Design review of the part built by this model. Coordinates are the model's own, in mm. Face numbers are marked on the shaded views. A direction names the side the tool comes from. Give positions to 0.01 mm unless a question says otherwise; leave off trailing zeros. Write each loop counter-clockwise with the first axis right and the second up, starting at its lowest first coordinate (ties: lowest second). Pieces come first, ordered by that corner, then holes.
```python
from build123d import *

# Parameters (mm, degrees)
BOTTOM_SKETCH_W                   = 101.6
BOTTOM_SKETCH_H                   = 76.2
BASE_EXTRUDE_DEPTH                = 12.7
CORNER_FILLETS_R                  = 12.7
TOP_CIRCULAR_SKETCH_R             = 5.5626
TOP_CIRCULAR_CUT_DEPTH            = 6.35
BOTTOM_CIRCULAR_SKETCH_R          = 3.3782
BOTTOM_CIRCULAR_CUT_DEPTH         = 64.816710194
HORIZONTAL_MIRROR_COPY_1_SKETCH_R = 5.5626
HORIZONTAL_MIRROR_COPY_1_DEPTH    = 6.35
HORIZONTAL_MIRROR_COPY_2_SKETCH_R = 3.3782
HORIZONTAL_MIRROR_COPY_2_DEPTH    = 64.816710194
OCTAGONAL_EXTRUDE_REACH           = 108.471
CENTER_SKETCH_R                   = 7.9375
CENTER_CUT_DEPTH                  = 110.090169628
RADIUS_SKETCH_R                   = 4.7752


with BuildPart() as part:
    # Bottom Sketch → Base Extrude (new body)
    with BuildSketch(Plane(origin=(0, 0, 0), x_dir=(1, 0, 0), z_dir=(0, 1, 0))):
        Rectangle(BOTTOM_SKETCH_W, BOTTOM_SKETCH_H)
    extrude(amount=BASE_EXTRUDE_DEPTH)

    # Corner Fillets
    corner_fillets_edges = [part.edges().sort_by_distance(p)[0] for p in [
        (-50.8, 6.35, -38.1),
        (50.8, 6.35, -38.1),
        (50.8, 6.35, 38.1),
        (-50.8, 6.35, 38.1),
    ]]
    fillet(corner_fillets_edges, radius=CORNER_FILLETS_R)

    # Top Circular Sketch → Top Circular Cut (cut)
    with BuildSketch(Plane(origin=(0, 12.7, 0), x_dir=(1, 0, 0), z_dir=(0, 1, 0))):
        with Locations(Location((-38.1, -25.4, 0), (0, 0, 270))):
            Circle(TOP_CIRCULAR_SKETCH_R)
    top_circular_cut = extrude(amount=-TOP_CIRCULAR_CUT_DEPTH, mode=Mode.SUBTRACT)

    # Bottom Circular Sketch → Bottom Circular Cut (cut, through all)
    with BuildSketch(Plane(origin=(0, 6.35, 0), x_dir=(1, 0, 0), z_dir=(0, 1, 0))):
        with Locations(Location((-38.1, -25.4, 0), (0, 0, 270))):
            Circle(BOTTOM_CIRCULAR_SKETCH_R)
    bottom_circular_cut = extrude(amount=-BOTTOM_CIRCULAR_CUT_DEPTH, mode=Mode.SUBTRACT)

    # Vertical Mirror: Top Circular Cut, Bottom Circular Cut across plane
    add(top_circular_cut.mirror(Plane.XY), mode=Mode.SUBTRACT)
    add(bottom_circular_cut.mirror(Plane.XY), mode=Mode.SUBTRACT)

    # Horizontal Mirror: Top Circular Cut, Bottom Circular Cut across plane
    add(top_circular_cut.mirror(Plane(origin=(0, 0, 0), x_dir=(0, 0, 1), z_dir=(1, 0, 0))), mode=Mode.SUBTRACT)
    add(bottom_circular_cut.mirror(Plane(origin=(0, 0, 0), x_dir=(0, 0, 1), z_dir=(1, 0, 0))), mode=Mode.SUBTRACT)

    # Horizontal Mirror copy 1 sketch → Horizontal Mirror copy 1 (cut)
    with BuildSketch(Plane(origin=(0, 12.7, 0), x_dir=(-1, 0, 0), z_dir=(0, 1, 0))):
        with Locations(Location((-38.1, -25.4, 0), (0, 0, 270))):
            Circle(HORIZONTAL_MIRROR_COPY_1_SKETCH_R)
    extrude(amount=-HORIZONTAL_MIRROR_COPY_1_DEPTH, mode=Mode.SUBTRACT)

    # Horizontal Mirror copy 2 sketch → Horizontal Mirror copy 2 (cut, through all)
    with BuildSketch(Plane(origin=(0, 6.35, 0), x_dir=(-1, 0, 0), z_dir=(0, 1, 0))):
        with Locations(Location((-38.1, -25.4, 0), (0, 0, 270))):
            Circle(HORIZONTAL_MIRROR_COPY_2_SKETCH_R)
    extrude(amount=-HORIZONTAL_MIRROR_COPY_2_DEPTH, mode=Mode.SUBTRACT)

    # Octagonal Extrude: up to this plane
    octagonal_extrude_end = Plane(origin=(0, 12.7, 0), z_dir=(0, 1, 0))
    # Octagonal Sketch → Octagonal Extrude (add, up to the surface)
    with BuildSketch(Plane(origin=(35.921024484, 48.621024484, 0), x_dir=(0.7071067811865488, -0.7071067811865462, 0), z_dir=(0.7071067811865462, 0.7071067811865488, 0)), mode=Mode.PRIVATE) as octagonal_extrude_sk1:
        Polygon((-7.290119387, 17.599905094), (-17.599905094, 7.290119387), (-17.599905094, -7.290119387), (-7.290119387, -17.599905094), (7.290119387, -17.599905094), (17.599905094, -7.290119387), (17.599905094, 7.290119387), (7.290119387, 17.599905094), align=None)
    octagonal_extrude_tool1 = split(extrude(octagonal_extrude_sk1.sketch, amount=-OCTAGONAL_EXTRUDE_REACH, mode=Mode.PRIVATE), bisect_by=octagonal_extrude_end, keep=Keep.BOTH, mode=Mode.PRIVATE)
    add(octagonal_extrude_tool1.solids().sort_by_distance((35.921024, 48.621024, 0))[0])

    # Center Sketch → Center Cut (cut, through all)
    with BuildSketch(Plane(origin=(42.271024484, 42.271024484, 0), x_dir=(0, 0, -1), z_dir=(0.7071067811865465, 0.7071067811865487, 0))):
        with Locations(Location((0, 8.980256121, 0), (0, 0, 90))):
            Circle(CENTER_SKETCH_R)
    extrude(amount=-CENTER_CUT_DEPTH, mode=Mode.SUBTRACT)

    # Radius Sketch → Radial Cut (revolve, cut)
    with BuildSketch(Plane(origin=(-6.35, 6.35, 0), x_dir=(0, 0, 1), z_dir=(-0.7071067811865478, 0.7071067811865472, 0)), mode=Mode.PRIVATE) as radial_cut_sk:
        with Locations((17.599905094, 40.730256121)):
            Circle(RADIUS_SKETCH_R)
    revolve(radial_cut_sk.sketch.rotate(Axis((0, 12.7, 0), (0.7071067811865462, 0.7071067811865488, 0)), 67.500000005), axis=Axis((0, 12.7, 0), (0.7071067811865462, 0.7071067811865488, 0)), mode=Mode.SUBTRACT)


solid = part.part
```
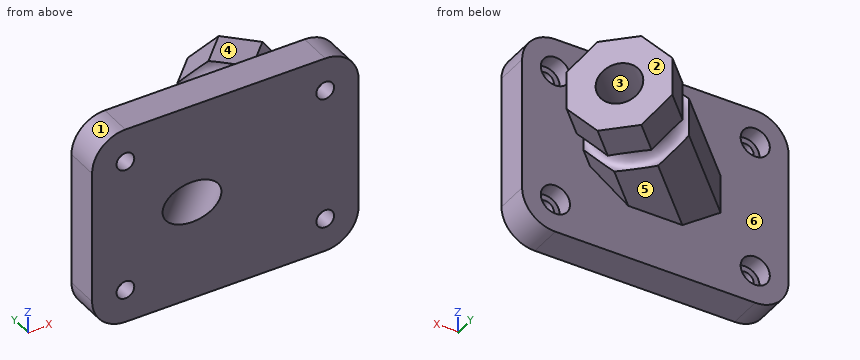
(1) To check wall thickness, follow L1, parallel to Z at x = 38.1, y = 8.75; L2, parallel to X at y = 4.5, z = -25.4; L3, parallel to Z at x = -38, y = 4. State the ranges of each line that lie inside material, in increasing order.
Resolved:
L1: z = -38.1 to -30.96, -19.84 to 19.84, 30.96 to 38.1
L2: x = -50.8 to -41.48, -34.72 to 34.72, 41.48 to 50.8
L3: z = -38.1 to -28.78, -22.02 to 22.02, 28.78 to 38.1
(2) Clearance check with flat-ended pins moving along their axes: P1, Ø3, axis at x = -28.5, z = 14.5, coming from the +Y side; P2, Ø16.5, axis at x = 33.5, y = 46, coming from the -Z side; P3, Ø6, axis at x = 33, y = 46, coming from the +Z side. State where each tip first meets the part, or that it passes through.
Resolved:
P1: stops at y = 12.7
P2: stops at z = -17.6
P3: stops at z = 17.6
(3) Tool access review of the marked faces 4, 5 and 6: name each direction out of +Z, -Z, +X, -X, +Y, -Y from which nothing blocks a thin tool from reaching the whole face with its end or side.
Resolved:
face 4: +Z, +X, -X, +Y
face 5: -Z, +X, -X, +Y
face 6: none
(4) Consider section B-B, the plane y = 8. Give the number of separate pieces and of enclosed holes in the cut face, then the cut area to 3 significant figures.
Resolved:
separate pieces: 1
enclosed holes: 5
area: 6,930 mm2
(5) Consider section A-A, the plane x = -36.5. Give the boundary of the cut face in (y, z), then the cut area to 3 significant figures.
Resolved:
outline: (0, -38.1) - (12.7, -38.1) - (12.7, -30.73) - (6.35, -30.73) - (6.35, -28.38) - (0, -28.38) - close; (0, -22.42) - (6.35, -22.42) - (6.35, -20.07) - (12.7, -20.07) - (12.7, 20.07) - (6.35, 20.07) - (6.35, 22.42) - (0, 22.42) - close; (0, 28.38) - (6.35, 28.38) - (6.35, 30.73) - (12.7, 30.73) - (12.7, 38.1) - (0, 38.1) - close
area: 757 mm2
(6) Mouldability with a two-part tool opening along Y and no side actions: class the marked faces 1, 2 and 3 as pulls with the +Y half, pulls with the -Y half, needs draft (parallel to the pull), parting line crosses it, or undercut.
Resolved:
face 1: needs draft
face 2: pulls with the +Y half
face 3: undercut
